Verification items for the finished model (mm, model axes). Coordinates: 2 decimals unless noted, no trailing zeros. Write each loop counter-clockwise with the first axis right and the second up, starting at its lowest first coordinate (ties: lowest second). Pieces come first, ordered by that corner, then holes. Notation, with made-up numbers: (77.5, 39) -> (93.5, 39) arc R12 ccw to (93.5, 55) -> close; hole circle Ø3 at (36, 33.5). An arc over 180 degrees is marked (long way). Answer in a Markdown table with one row per item.
```python
from build123d import *

# Parameters (mm, degrees)
EXTRUDE1_DEPTH = 177.8
FILLET1_R      = 63.5
FILLET2_R      = 25.4


with BuildPart() as part:
    # Sketch1 → Extrude1 (new body)
    with BuildSketch(Plane.XY):
        Polygon((0, 152.4), (0, 0), (295.275, 0), (295.275, 38.1), (228.6, 50.8), (133.35, 95.25), (66.675, 152.4), align=None)
    extrude(amount=-EXTRUDE1_DEPTH)

    # Fillet1
    fillet1_edges = [part.edges().sort_by_distance(p)[0] for p in [
        (228.6, 50.8, -88.9),
        (66.675, 152.4, -88.9),
        (133.35, 95.25, -88.9),
    ]]
    fillet(fillet1_edges, radius=FILLET1_R)

    # Fillet2
    fillet2_edges = [part.edges().sort_by_distance(p)[0] for p in [
        (0, 76.2, -177.8),
        (0, 76.2, 0),
    ]]
    fillet(fillet2_edges, radius=FILLET2_R)


solid = part.part
```
1. Go/stop test with flat-tipped pins: pin 1 (8 mm diameter, centred on x = 138, z = -65, fed in from +Y); pin 2 (5 mm diameter, centred on x = 220, z = -21.5, fed in from +Y); pin 3 (2 mm diameter, centred on y = 101, z = -119.5, fed in from +X). Record where each tip stops, or that it passes through.
Findings below:
| item | result |
|---|---|
| pin 1 | stops at y = 95.54 |
| pin 2 | stops at y = 55.98 |
| pin 3 | stops at x = 127.83 |
2. Sectioned sample at C-C, the plane x = 162. Record the cut outline in (y, z).
Findings below:
| item | result |
|---|---|
| outline | (0, -177.8) -> (81.88, -177.8) -> (81.88, 0) -> (0, 0) -> close |
3. Sectioned sample at A-A, the plane z = -142. Record the cut outline in (x, y) (1 decimal).
Findings below:
| item | result |
|---|---|
| outline | (0, 0) -> (295.3, 0) -> (295.3, 38.1) -> (236.4, 49.3) arc R63.5 cw to (221.4, 54.2) -> (141.2, 91.6) arc R63.5 cw to (126.8, 100.9) -> (84.5, 137.1) arc R63.5 ccw to (43.2, 152.4) -> (0, 152.4) -> close |
4. Material ranges on probe 1 along Y at (x, z) = (45, -50); probe 2 along X at (y, z) = (90.5, -53); probe 3 along Y at (x, z) = (236.5, -79), recorded low to high. Write a range as from..to.
Findings below:
| item | result |
|---|---|
| probe 1 | y = 0..152.37 |
| probe 2 | x = 0..143.53 |
| probe 3 | y = 0..49.3 |
5. Sectioned sample at D-D, the plane z = -165.5. Record the cut outline in (x, y) (1 decimal).
Findings below:
| item | result |
|---|---|
| outline | (3.6, 0) -> (295.3, 0) -> (295.3, 38.1) -> (236.4, 49.3) arc R63.5 cw to (221.4, 54.2) -> (141.2, 91.6) arc R63.5 cw to (126.8, 100.9) -> (84.5, 137.1) arc R63.5 ccw to (43.2, 152.4) -> (3.6, 152.4) -> close |
6. Sectioned sample at B-B, the plane y = 76. Record the cut outline in (x, z).
Findings below:
| item | result |
|---|---|
| outline | (0, -152.4) arc R25.4 ccw to (25.4, -177.8) -> (174.6, -177.8) -> (174.6, 0) -> (25.4, 0) arc R25.4 ccw to (0, -25.4) -> close |
